Geometry check sheet. Reference: the model listing, model coordinates, mm. A direction names the side the tool comes from. Coordinates: 2 decimals unless noted, no trailing zeros. Write each loop counter-clockwise with the first axis right and the second up, starting at its lowest first coordinate (ties: lowest second). Pieces come first, ordered by that corner, then holes. Notation, with made-up numbers: (64, 74.25) -> (97, 74.25) arc R19 ccw to (97, 89.25) -> close; hole circle Ø11 at (18, 66). An arc over 180 degrees is marked (long way). One line per question, with ' | ' between items.
```python
from build123d import *

# Parameters (mm, degrees)
SKETCH1_W                   = 62.865
SKETCH1_H                   = 71.12
BOSS_EXTRUDE1_DEPTH         = 20.6248
CUT_EXTRUDE2_DEPTH          = 52.748410906
CUT_EXTRUDE2_DEPTH_BACK     = 52.748410906
SKETCH4_R                   = 3.175
FILLET1_R                   = 2.54
SKETCH2_W                   = 35.433
SKETCH2_H                   = 43.688
CUT_EXTRUDE3_DEPTH          = 68.839744016
SKETCH6_R                   = 2.7686
CUT_EXTRUDE4_DEPTH          = 27.94
SKETCH7_R                   = 10.3124
BOSS_EXTRUDE2_DEPTH         = 17.78
CUT_EXTRUDE5_START          = -17.78
CUT_EXTRUDE5_DEPTH          = 17.78
SKETCH9_R                   = 4.7625
CUT_EXTRUDE6_DEPTH          = 3.175
F_1_2_20_TAPPED_HOLE1_D     = 11.50874
F_1_2_20_TAPPED_HOLE1_DEPTH = 28.321


with BuildPart() as part:
    # Sketch1 → Boss-Extrude1 (new body)
    with BuildSketch(Plane.XY):
        Rectangle(SKETCH1_W, SKETCH1_H)
    extrude(amount=BOSS_EXTRUDE1_DEPTH)

    # Sketch4 → Cut-Extrude2 (cut, two sides: drawn at the far end of the back side and taken through both)
    with BuildSketch(Plane.XY.offset(20.6248).offset(-CUT_EXTRUDE2_DEPTH_BACK)):
        with Locations((-12.7, 29.21)):
            Circle(SKETCH4_R)
        with Locations((-25.4, 15.875)):
            Circle(SKETCH4_R)
        with Locations((-12.7, -29.21)):
            Circle(SKETCH4_R)
        with Locations((-25.4, -15.875)):
            Circle(SKETCH4_R)
        with Locations((12.7, -29.21)):
            Circle(SKETCH4_R)
        with Locations((12.7, 29.21)):
            Circle(SKETCH4_R)
        with Locations((25.4, 0)):
            Circle(SKETCH4_R)
        with Locations((25.4, 22.225)):
            Circle(SKETCH4_R)
        with Locations((25.4, -22.225)):
            Circle(SKETCH4_R)
    extrude(amount=CUT_EXTRUDE2_DEPTH + CUT_EXTRUDE2_DEPTH_BACK, mode=Mode.SUBTRACT)

    # Sketch5 → Revolve2 (revolve)
    with BuildSketch(Plane(origin=(0, 0, 0), x_dir=(0, 0, -1), z_dir=(1, 0, 0)), mode=Mode.PRIVATE) as revolve2_sk:
        with BuildLine():
            Line((-16.6624, 35.56), (-16.6624, 50.119871939))
            ThreePointArc((-16.6624, 50.119871939), (-14.802528061, 54.61), (-10.3124, 56.469871939))
            Line((-10.3124, 56.469871939), (-10.3124, 35.56))
            Line((-10.3124, 35.56), (-16.6624, 35.56))
        make_face()
    revolve(revolve2_sk.sketch.rotate(Axis((0, 35.56, 10.3124), (0, 1, 0)), 180), axis=Axis((0, 35.56, 10.3124), (0, 1, 0)))

    # Fillet1
    fillet1_edges = [part.edges().sort_by_distance(p)[0] for p in [
        (0, 35.56, 16.6624),
    ]]
    fillet(fillet1_edges, radius=FILLET1_R)

    # Sketch2 → Cut-Extrude3 (cut, through all)
    with BuildSketch(Plane.XY.offset(20.6248)):
        Rectangle(SKETCH2_W, SKETCH2_H)
    extrude(amount=-CUT_EXTRUDE3_DEPTH, mode=Mode.SUBTRACT)

    # Sketch6 → Cut-Extrude4 (cut)
    with BuildSketch(Plane.XZ.offset(-21.844)):
        with Locations(Location((0, 10.3124, 0), (0, 0, 270))):
            Circle(SKETCH6_R)
    extrude(amount=-CUT_EXTRUDE4_DEPTH, mode=Mode.SUBTRACT)

    # Sketch7 → Boss-Extrude2 (add)
    with BuildSketch(Plane.XZ.offset(35.56)):
        with Locations(Location((0, 10.3124, 0), (0, 0, 270))):
            Circle(SKETCH7_R)
    extrude(amount=BOSS_EXTRUDE2_DEPTH)

    # Sketch8 → Cut-Extrude5 (cut)
    with BuildSketch(Plane.XZ.offset(53.34).offset(CUT_EXTRUDE5_START)):
        with BuildLine():
            Line((-7.399596954, 3.12967359), (-5.795378061, 3.12967359))
            Line((-5.795378061, 3.12967359), (7.399596954, 3.12967359))
            ThreePointArc((7.399596954, 3.12967359), (0, 0), (-7.399596954, 3.12967359))
        make_face()
    extrude(amount=CUT_EXTRUDE5_DEPTH, mode=Mode.SUBTRACT)

    # Sketch9 → Cut-Extrude6 (cut)
    with BuildSketch(Plane(origin=(0, -21.844, 0), x_dir=(1, 0, 0), z_dir=(0, 1, 0))):
        with Locations(Location((0, -10.3124, 0), (0, 0, 270))):
            Circle(SKETCH9_R)
    extrude(amount=-CUT_EXTRUDE6_DEPTH, mode=Mode.SUBTRACT)

    # 1/2-20 Tapped Hole1
    with Locations(Plane(origin=(0, -53.34, 0), x_dir=(-1, 0, 0), z_dir=(0, -1, 0))):
        with Locations((0, -10.3124)):
            Hole(F_1_2_20_TAPPED_HOLE1_D / 2, depth=F_1_2_20_TAPPED_HOLE1_DEPTH)


solid = part.part
```
(1) Cross-section at D-D (y = -8.5). Record the cut outline in (x, z).
Answers below:
outline: (-31.43, 0) -> (-17.72, 0) -> (-17.72, 20.62) -> (-31.43, 20.62) -> close; (17.72, 0) -> (31.43, 0) -> (31.43, 20.62) -> (17.72, 20.62) -> close
(2) Tool access check on faces 1 (the face through (0, -44, 3.13)), 2 (the face through (-21, 0, 0)), 3 (the face through (0, 49.784, 10)), 4 (the face through (-4, -21.844, 15)). Record the directions out of +Z, -Z, +X, -X, +Y, -Y that give a thin tool (end or side, any length) a straight path to the whole face; none if there is none.
Answers below:
face 1: -Z, +X, -X, -Y | face 2: -Z, +X, -X, +Y, -Y | face 3: -Y | face 4: +Z, -Z
(3) Cross-section at C-C (x = -25.4). Record the cut outline in (y, z), plus the area to 3 significant figures.
Answers below:
outline: (-35.56, 0) -> (-19.05, 0) -> (-19.05, 20.62) -> (-35.56, 20.62) -> close; (-12.7, 0) -> (12.7, 0) -> (12.7, 20.62) -> (-12.7, 20.62) -> close; (19.05, 0) -> (35.56, 0) -> (35.56, 20.62) -> (19.05, 20.62) -> close | area: 1,200 mm²
(4) Draft check along X on faces 5 (the face through (-22.37, 16.83, 10.17)), 6 (the face through (-21, 0, 20.625)), 7 (the face through (31.432, 0, 10)). Enter one of: pulls with the +X half, pulls with the -X half, needs draft (parallel to the pull), parting line crosses it, or undercut.
Answers below:
face 5: undercut | face 6: needs draft | face 7: pulls with the +X half
(5) Cross-section at B-B (x = -12.7). Record the cut outline in (y, z) (3 decimals), plus the area to 3 significant figures.
Answers below:
outline: (-35.56, 0) -> (-32.385, 0) -> (-32.385, 20.625) -> (-35.56, 20.625) -> close; (-26.035, 0) -> (-21.844, 0) -> (-21.844, 20.625) -> (-26.035, 20.625) -> close; (21.844, 0) -> (26.035, 0) -> (26.035, 20.625) -> (21.844, 20.625) -> close; (32.385, 0) -> (35.56, 0) -> (35.56, 20.625) -> (32.385, 20.625) -> close | area: 304 mm²
(6) Depth check by flat-ended pin: P1, Ø5, axis at x = -13.5, z = 4, coming from the -Y side; P2, Ø10, axis at x = 12.7, y = -29.21, coming from the -Z side; P3, Ø10.5, axis at x = 0, z = 10.31, coming from the -Y side; P4, Ø6, axis at x = -7.5, z = 8, coming from the +Y side. Enter the tip coordinate at first touch or a pass-through.
Answers below:
P1: stops at y = -35.56 | P2: stops at z = 0 | P3: stops at y = -25.02 | P4: stops at y = 54.22
(7) Cross-section at A-A (y = 29.21). Record the cut outline in (x, z) (1 decimal).
Answers below:
outline: (-31.4, 0) -> (-15.9, 0) -> (-15.9, 20.6) -> (-31.4, 20.6) -> close; (-9.5, 0) -> (9.5, 0) -> (9.5, 20.6) -> (-9.5, 20.6) -> close; (15.9, 0) -> (31.4, 0) -> (31.4, 20.6) -> (15.9, 20.6) -> close; hole circle Ø5.5 at (0, 10.3)
(8) Material ranges on line 1 (Y direction, x = 25.4, z = 6.75) (3 decimals); line 2 (Y direction, x = 12.7, z = 5.5) (3 decimals); line 3 (X direction, y = 29.21, z = 14.75) (1 decimal), recorded low to high.
Answers below:
line 1: y = -35.56 to -25.4, -19.05 to -3.175, 3.175 to 19.05, 25.4 to 35.56 | line 2: y = -35.56 to -32.385, -26.035 to -21.844, 21.844 to 26.035, 32.385 to 35.56 | line 3: x = -31.4 to -15.9, -9.5 to 9.5, 15.9 to 31.4
